from build123d import *

# Parameters (mm, degrees)
SKETCH1_W                                       = 2.45
SKETCH1_H                                       = 9
BOSS_EXTRUDE1_DEPTH                             = 13.5
BOSS_EXTRUDE2_DEPTH                             = 0.6
BOSS_EXTRUDE3_START                             = -13.5
SKETCH1_4_W                                     = 2.45
SKETCH1_4_H                                     = 9
BOSS_EXTRUDE3_DEPTH                             = 1
MIRROR1_START                                   = -13.5
MIRROR1_OUTLINE_R                               = 6.25
MIRROR1_DEPTH                                   = 13.5
MIRROR1_START_2                                 = -0.6
MIRROR1_2_OUTLINE_R                             = 6.25
MIRROR1_2_DEPTH                                 = 0.6
MIRROR1_START_3                                 = -14.5
MIRROR1_3_DEPTH                                 = 1
CSK_FOR_M5_FLAT_HEAD_MACHINE_SCREW1_D           = 5.3
CSK_FOR_M5_FLAT_HEAD_MACHINE_SCREW1_CSINK_D     = 10.4
CSK_FOR_M5_FLAT_HEAD_MACHINE_SCREW1_CSINK_ANGLE = 90


# Read off the part's stored shape, not the designer's step: Mirror1
with BuildPart() as part:
    # Sketch1 → Boss-Extrude1 (new body)
    with BuildSketch(Plane(origin=(0, 0, 0), x_dir=(1, 0, 0), z_dir=(0, 1, 0))):
        with Locations((1.225, 4.5)):
            Rectangle(SKETCH1_W, SKETCH1_H)
        with BuildLine():
            Line((2.45, 9), (2.45, 0))
            Line((2.45, 0), (6.25, 0))
            ThreePointArc((6.25, 0), (12.5, 6.25), (18.75, 0))
            Line((18.75, 0), (21.5, 0))
            ThreePointArc((21.5, 0), (18.863961031, 6.363961031), (12.5, 9))
            Line((12.5, 9), (2.45, 9))
        make_face()
    extrude(amount=-BOSS_EXTRUDE1_DEPTH)

    # Sketch1<3> → Boss-Extrude2 (add)
    with BuildSketch(Plane(origin=(0, 0, 0), x_dir=(1, 0, 0), z_dir=(0, 1, 0))):
        with BuildLine():
            ThreePointArc((18.75, 0), (12.5, 6.25), (6.25, 0))
            Line((6.25, 0), (18.75, 0))
        make_face()
    extrude(amount=-BOSS_EXTRUDE2_DEPTH)

    # Sketch1<4> → Boss-Extrude3 (add)
    with BuildSketch(Plane(origin=(0, 0, 0), x_dir=(1, 0, 0), z_dir=(0, 1, 0)).offset(BOSS_EXTRUDE3_START)):
        with Locations((1.225, 4.5)):
            Rectangle(SKETCH1_4_W, SKETCH1_4_H)
    extrude(amount=-BOSS_EXTRUDE3_DEPTH)

    # Mirror1 outline → Mirror1 (add)
    with BuildSketch(Plane(origin=(0, 0, 0), x_dir=(1, 0, 0), z_dir=(0, 1, 0)).offset(MIRROR1_START)):
        with BuildLine():
            Line((21.5, 0), (18.75, 0))
            ThreePointArc((18.75, 0), (12.5, -6.25), (6.25, 0))
            Line((6.25, 0), (0, 0))
            Line((0, 0), (0, 9))
            Line((0, 9), (-12.5, 9))
            ThreePointArc((-12.5, 9), (-21.5, 0), (-12.5, -9))
            Line((-12.5, -9), (12.5, -9))
            ThreePointArc((12.5, -9), (18.863961031, -6.363961031), (21.5, 0))
        make_face()
        with Locations((-12.5, 0)):
            Circle(MIRROR1_OUTLINE_R, mode=Mode.SUBTRACT)
    extrude(amount=MIRROR1_DEPTH)

    # Mirror1 2 outline → Mirror1 2 (add)
    with BuildSketch(Plane(origin=(0, 0, 0), x_dir=(1, 0, 0), z_dir=(0, 1, 0)).offset(MIRROR1_START_2)):
        with BuildLine():
            ThreePointArc((6.25, 0), (12.5, -6.25), (18.75, 0))
            Line((18.75, 0), (6.25, 0))
        make_face()
        with Locations((-12.5, 0)):
            Circle(MIRROR1_2_OUTLINE_R)
    extrude(amount=MIRROR1_2_DEPTH)

    # Mirror1 3 outline → Mirror1 3 (add)
    with BuildSketch(Plane(origin=(0, 0, 0), x_dir=(1, 0, 0), z_dir=(0, 1, 0)).offset(MIRROR1_START_3)):
        Polygon((2.45, -9), (2.45, 0), (0, 0), (0, 9), (-2.45, 9), (-2.45, -9), align=None)
    extrude(amount=MIRROR1_3_DEPTH)

    # CSK for M5 Flat Head Machine Screw1 (through all)
    with Locations(Plane(origin=(0, 0, 0), x_dir=(1, 0, 0), z_dir=(0, 1, 0))):
        with Locations((0, 0)):
            CounterSinkHole(CSK_FOR_M5_FLAT_HEAD_MACHINE_SCREW1_D / 2, CSK_FOR_M5_FLAT_HEAD_MACHINE_SCREW1_CSINK_D / 2, counter_sink_angle=CSK_FOR_M5_FLAT_HEAD_MACHINE_SCREW1_CSINK_ANGLE)


solid = part.part
Read the model definition and answer for the solid it produces. Units are mm, in the model's axes. A direction names the side the tool comes from. Coordinates: 2 decimals unless noted, no trailing zeros. Loops run counter-clockwise (first coordinate to the right, second up) from the corner with the lowest first, then second, coordinate; pieces in that order, holes last. Notation, with made-up numbers: (53, 78) - (94, 78) arc R20 ccw to (94, 109) - close; hole circle Ø4 at (83, 10). An arc over 180 degrees is marked (long way). Answer in a Markdown table with one row per item.
Q1. The mould has two halves that part along X. Classify faces 1 (the flat face through (0, -14.5, -6)), 2 (the flat face through (-2.45, -14, -5)), 3 (the flat face through (2.45, -14, 5)), 4 (the conical face through (0.601, -2.426, 2.708)): pulls with the +X half, pulls with the -X half, needs draft (parallel to the pull), parting line crosses it, or undercut.
Here are the results:
| item | result |
|---|---|
| face 1 | needs draft |
| face 2 | pulls with the -X half |
| face 3 | pulls with the +X half |
| face 4 | undercut |
Q2. Find section C-C on z = 8.25. Write down the section's boundary in (x, y), plus the area to 3 significant figures.
Here are the results:
| item | result |
|---|---|
| outline | (-16.1, -13.5) - (-2.45, -13.5) - (-2.45, -14.5) - (2.45, -14.5) - (2.45, -13.5) - (16.1, -13.5) - (16.1, 0) - (-16.1, 0) - close |
| area | 440 mm^2 |
Q3. Find section B-B on y = -7.5. Write down the section's boundary in (x, z), plus the area to 3 significant figures.
Here are the results:
| item | result |
|---|---|
| outline | (-12.5, -9) - (12.5, -9) arc R9 ccw to (12.5, 9) - (-12.5, 9) arc R9 ccw to start; hole circle Ø12.5 at (-12.5, 0); hole circle Ø5.3 at (0, 0); hole circle Ø12.5 at (12.5, 0) |
| area | 437 mm^2 |
Q4. Find section A-A on x = 0. Write down the section's boundary in (y, z).
Here are the results:
| item | result |
|---|---|
| outline | (-14.5, -9) - (0, -9) - (0, -5.2) - (-2.55, -2.65) - (-14.5, -2.65) - close; (-14.5, 2.65) - (-2.55, 2.65) - (0, 5.2) - (0, 9) - (-14.5, 9) - close |
Q5. For faces 5 (the flat face through (-6, -13.5, 0)), 6 (the flat face through (-13, -0.6, 0)), 7 (the flat face through (2.45, -14, -5)), determine the directions among +Z, -Z, +X, -X, +Y, -Y from which every point of the face is accessible in a straight line to the end or side of a thin tool.
Here are the results:
| item | result |
|---|---|
| face 5 | +Z, -Z, -X, -Y |
| face 6 | -Y |
| face 7 | +Z, -Z, +X, -Y |
Q6. Straight lines are drawn through the part: line 1 along Z through (x, y) = (0, -7); line 2 along Z through (x, y) = (-12.5, -9.25); line 3 along X through (y, z) = (-1.25, 3). For each, find the intervals that lie inside material, in ascending order. Write a range as [from, to].
Here are the results:
| item | result |
|---|---|
| line 1 | z = [-9, -2.65], [2.65, 9] |
| line 2 | z = [-9, -6.25], [6.25, 9] |
| line 3 | x = [-20.99, -17.98], [-7.02, -2.57], [2.57, 7.02], [17.98, 20.99] |
Q7. Given P1, Ø10, axis at x = -12.5, z = -2.5, coming from the -Y side; P2, Ø1, axis at y = -11.5, z = 3.5, coming from the +X side; P3, Ø0.8, axis at y = -14, z = -4, coming from the +X side; P4, Ø3, axis at x = 0, z = 0, coming from the +Y side, each flat-ended and moving along its own axis, determine where each tip first touches the part or whether it passes through.
Here are the results:
| item | result |
|---|---|
| P1 | stops at y = -13.5 |
| P2 | stops at x = 20.99 |
| P3 | stops at x = 2.45 |
| P4 | passes through |
